```python
from build123d import *

# Parameters (mm, degrees)
F0_W     = 129.54
F0_H     = 129.54
F1_DEPTH = 57.15
F2_T     = -3.175
F3_R     = 1.524
F4_R     = 1.524
F5_W     = 3.175
F5_H     = 1.524
F5_H_2   = 120.142
F6_DEPTH = 53.975
F7_R     = 1.524


with BuildPart() as f1:
    # F0 (on Front) → F1 (new body)
    with BuildSketch(Plane.XZ):
        with Locations((64.77, 64.77)):
            Rectangle(F0_W, F0_H)
    extrude(amount=-F1_DEPTH)

    # F2
    f2_openings = [f1.faces().sort_by_distance(p)[0] for p in [
        (64.77, 0, 64.77),
    ]]
    offset(amount=F2_T, openings=f2_openings)

    # F3
    f3_edges = [f1.edges().sort_by_distance(p)[0] for p in [
        (3.175, 26.9875, 126.365),
        (64.77, 53.975, 126.365),
        (3.175, 53.975, 64.77),
        (3.175, 26.9875, 3.175),
        (64.77, 53.975, 3.175),
        (126.365, 53.975, 64.77),
        (126.365, 26.9875, 126.365),
        (126.365, 26.9875, 3.175),
    ]]
    fillet(f3_edges, radius=F3_R)

    # F4
    f4_edges = [f1.edges().sort_by_distance(p)[0] for p in [
        (129.54, 28.575, 0),
        (64.77, 57.15, 0),
        (129.54, 57.15, 64.77),
        (129.54, 28.575, 129.54),
        (64.77, 57.15, 129.54),
        (0, 28.575, 129.54),
        (0, 57.15, 64.77),
        (0, 28.575, 0),
    ]]
    fillet(f4_edges, radius=F4_R)

    # F5 (on face) → F6 (join)
    with BuildSketch(Plane.XZ.offset(-53.975)):
        with Locations((64.77, 125.603)):
            Rectangle(F5_W, F5_H)
        with Locations((64.77, 64.77)):
            Rectangle(F5_W, F5_H_2)
        with Locations((64.77, 3.937)):
            Rectangle(F5_W, F5_H)
    extrude(amount=F6_DEPTH)

    # F7
    f7_edges = [f1.edges().sort_by_distance(p)[0] for p in [
        (33.94075, 0, 126.365),
        (63.1825, 0, 64.77),
        (63.1825, 53.528631, 125.918631),
        (63.1825, 53.975, 64.77),
        (63.1825, 53.528631, 3.621369),
        (63.1825, 26.2255, 3.175),
        (63.1825, 26.2255, 126.365),
        (95.59925, 0, 126.365),
        (66.3575, 26.2255, 126.365),
        (95.59925, 52.451, 126.365),
        (124.841, 26.2255, 126.365),
        (126.365, 0, 64.77),
        (126.365, 26.2255, 4.699),
        (126.365, 26.2255, 124.841),
        (126.365, 52.451, 64.77),
        (3.175, 0, 64.77),
        (3.621369, 0, 125.918631),
        (33.94075, 0, 3.175),
        (3.621369, 0, 3.621369),
        (125.918631, 0, 125.918631),
        (125.918631, 0, 3.621369),
        (95.59925, 0, 3.175),
        (66.3575, 0, 64.77),
        (66.3575, 26.2255, 3.175),
        (66.3575, 53.528631, 3.621369),
        (66.3575, 53.975, 64.77),
        (66.3575, 53.528631, 125.918631),
    ]]
    fillet(f7_edges, radius=F7_R)


solid = f1.part
```
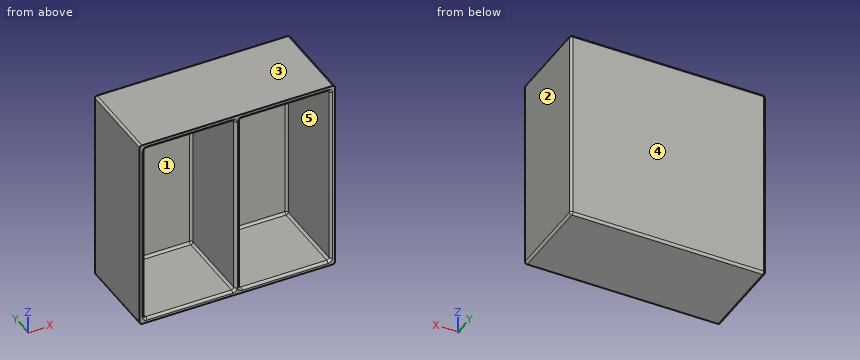
The model under review builds one solid part; all positions refer to its coordinate system, in mm. Face numbers are marked on the shaded views. A direction names the side the tool comes from. Round coordinates to 2 decimals unless told otherwise and drop trailing zeros. Loops run counter-clockwise (first coordinate to the right, second up) from the corner with the lowest first, then second, coordinate; pieces in that order, holes last. Notation, with made-up numbers: (-26, -2.5) - (11, -2.5) arc R22 ccw to (11, 25.5) - close; hole circle Ø11 at (30.25, 17). An arc over 180 degrees is marked (long way). Write each question's results on one line, items separated by ' | '. Start each with the question number.
Q1. Wall thickness on line 1 along X through (y, z) = (42, 98) (1 decimal); line 2 along Z through (x, y) = (42.5, 6) (3 decimals); line 3 along Y through (x, z) = (70.5, 18.5) (3 decimals): over which ranges is each line inside the solid? List them lowest first. Write a range as [from, to].
Q2. Take a section at A-A on y = 5. Give the boundary of the cut face in (x, z) (1 decimal).
Q3. Draft analysis for pull direction Z (two halves, no side actions). For the marked faces 1, 2 and 3, state which applies: pulls with the +Z half, pulls with the -Z half, needs draft (parallel to the pull), parting line crosses it, or undercut.
Q4. Take a section at C-C on x = 13. Give the boundary of the cut face in (y, z) (3 decimals), plus the area to 3 significant figures.
Q5. Tool access review of the marked faces 4 and 5: name each direction out of +Z, -Z, +X, -X, +Y, -Y from which nothing blocks a thin tool from reaching the whole face with its end or side.
Q6. Insertion check: P1, Ø6, axis at x = 83.5, z = 97.5, coming from the -Y side (3 decimals). The pin has a flat end and moves straight along its axis. Give the tip position at first contact, or say it passes through.
Data:
1) line 1: x = [0, 3.2], [63.2, 66.4], [126.4, 129.5] | line 2: z = [0, 3.175], [126.365, 129.54] | line 3: y = [53.975, 57.15]
2) outline: (0, 1.5) arc R1.5 ccw to (1.5, 0) - (128, 0) arc R1.5 ccw to (129.5, 1.5) - (129.5, 128) arc R1.5 ccw to (128, 129.5) - (1.5, 129.5) arc R1.5 ccw to (0, 128) - close; hole (3.2, 4.7) arc R1.5 ccw to (4.7, 3.2) - (61.7, 3.2) arc R1.5 ccw to (63.2, 4.7) - (63.2, 124.8) arc R1.5 ccw to (61.7, 126.4) - (4.7, 126.4) arc R1.5 ccw to (3.2, 124.8) - close; hole (66.4, 4.7) arc R1.5 ccw to (67.9, 3.2) - (124.8, 3.2) arc R1.5 ccw to (126.4, 4.7) - (126.4, 124.8) arc R1.5 ccw to (124.8, 126.4) - (67.9, 126.4) arc R1.5 ccw to (66.4, 124.8) - close
3) face 1: undercut | face 2: needs draft | face 3: pulls with the +Z half
4) outline: (0, 0) - (55.626, 0) arc R1.524 ccw to (57.15, 1.524) - (57.15, 128.016) arc R1.524 ccw to (55.626, 129.54) - (0, 129.54) - (0, 127.889) arc R1.524 ccw to (1.524, 126.365) - (52.451, 126.365) arc R1.524 cw to (53.975, 124.841) - (53.975, 4.699) arc R1.524 cw to (52.451, 3.175) - (1.524, 3.175) arc R1.524 ccw to (0, 1.651) - close | area: 753 mm²
5) face 4: +Z, -Z, +X, -X, +Y | face 5: -Y
6) P1: stops at y = 53.975
